Input: dimensioned drawing with shaded views. Units: mm. Origin: part minimum x, y, z. A direction names the side the tool comes from. Give positions to 0.01 mm unless a question says otherwise; leave off trailing zeros. Write each loop counter-clockwise with the first axis right and the second up, starting at its lowest first coordinate (ties: lowest second). Pieces come first, ordered by that corner, then holes. Notation, with made-up numbers: (21, 57) - (48, 57) arc R11 ccw to (48, 68) - close; hole circle Ø1 at (21.5, 45.25). An arc over 180 degrees is marked (long way). Answer as CSV lines item,"result".
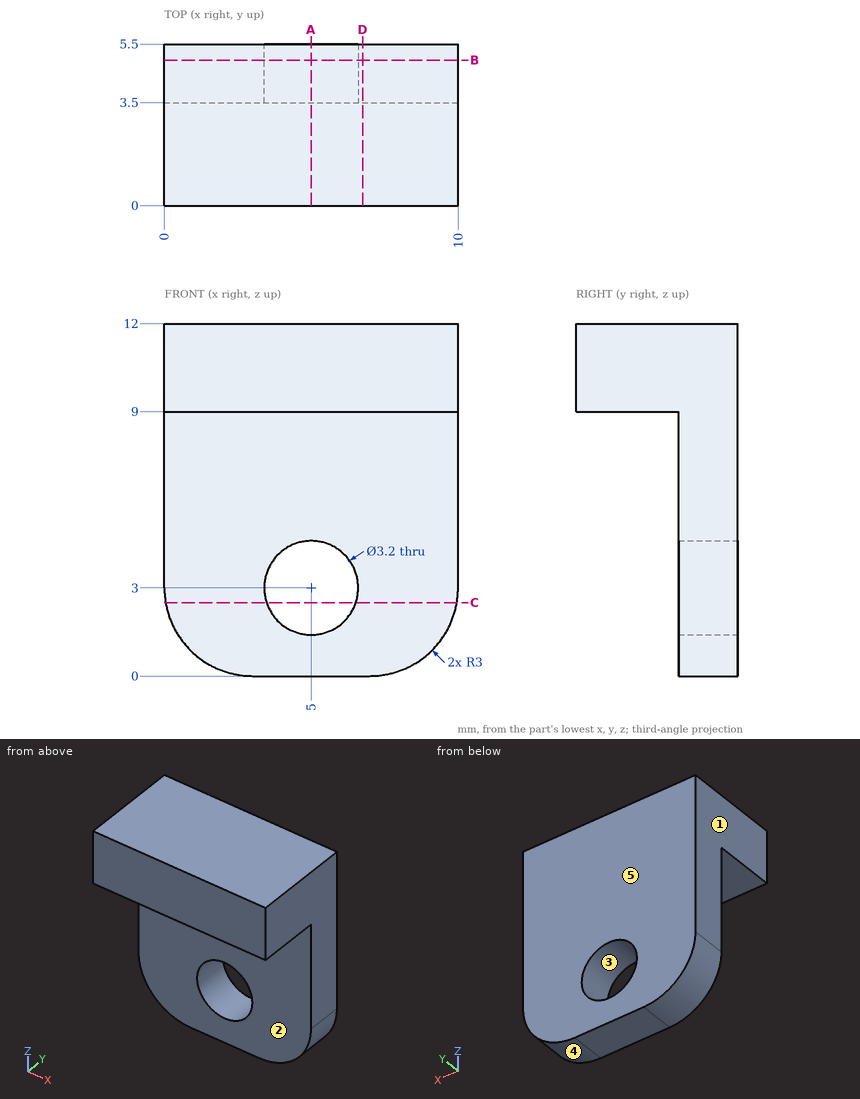
Item 1: Cut plane D-D on x = 6.75. Return the cut outline in (y, z), plus the area to 3 significant figures.
The answers:
outline,"(0, 9) - (3.5, 9) - (3.5, 0) - (5.5, 0) - (5.5, 12) - (0, 12) - close"
area,"34.5 mm²"
Item 2: Ray query, line 1 (Z direction, x = 5, y = 4.05); line 2 (Z direction, x = 4.5, y = 1.45); line 3 (Y direction, x = 7, z = 4.25). Return the intervals inside material, ascending. Write a range as from..to.
The answers:
line 1,"0..1.4, 4.6..12"
line 2,"9..12"
line 3,"3.5..5.5"
Item 3: Mould query, pull axis X, two halves, no side actions, for the marked faces 3, 4 and 5. Classes: +X half, -X half, draft (parallel to the pull), parting line (faces both ways), or undercut.
The answers:
face 3,"undercut"
face 4,"+X half"
face 5,"draft"
Item 4: Cut plane B-B on y = 4.95. Return the cut outline in (x, z), plus the area to 3 significant figures.
The answers:
outline,"(0, 3) arc R3 ccw to (3, 0) - (7, 0) arc R3 ccw to (10, 3) - (10, 12) - (0, 12) - close; hole circle Ø3.2 at (5, 3)"
area,"108 mm²"
Item 5: Contact query for flat-ended pins moving along their axis: pin 1 (5 mm diameter, centred on x = 4, z = 2.5, fed in from -Y); pin 2 (1.5 mm diameter, centred on x = 1.5, y = 1, fed in from -Z). Output: stop coordinate, or through.
The answers:
pin 1,"y = 3.5"
pin 2,"z = 9"
Item 6: Cut plane A-A on x = 5. Return the cut outline in (y, z).
The answers:
outline,"(0, 9) - (3.5, 9) - (3.5, 4.6) - (5.5, 4.6) - (5.5, 12) - (0, 12) - close; (3.5, 0) - (5.5, 0) - (5.5, 1.4) - (3.5, 1.4) - close"
Item 7: Cut plane C-C on z = 2.5. Return the cut outline in (x, y), plus the area to 3 significant figures.
The answers:
outline,"(0.04, 3.5) - (3.48, 3.5) - (3.48, 5.5) - (0.04, 5.5) - close; (6.52, 3.5) - (9.96, 3.5) - (9.96, 5.5) - (6.52, 5.5) - close"
area,"13.8 mm²"
Item 8: Reachability of the marked faces 1 and 2 from +Z, -Z, +X, -X, +Y, -Y: full face, straight path, thin tool, end or side. Return the list, or none.
The answers:
face 1,"+Z, -Z, -X, +Y, -Y"
face 2,"-Z, +X, -X, -Y"
